from build123d import *

# Parameters (mm, degrees)
F0_W     = 20
F0_H     = 20
F1_DEPTH = 15
F1_TAPER = 3
F2_R     = 2
F4_DEPTH = 3


with BuildPart() as f1:
    # F0 (on Top) → F1 (new body)
    with BuildSketch(Plane.XY):
        with Locations((0.5756109022, 1.4432906293)):
            Rectangle(F0_W, F0_H)
    extrude(amount=F1_DEPTH, taper=F1_TAPER)

    # F2
    f2_edges = [f1.edges().sort_by_distance(p)[0] for p in [
        (10.182552, 11.050232, 7.500009),
        (-9.031331, 11.050232, 7.5),
        (0.575611, 10.657174, 15),
        (9.789494, 1.443291, 15),
        (-8.638272, 1.443291, 15),
        (0.575611, -7.770593, 15),
        (10.182553, -8.163651, 7.5),
        (-9.031331, -8.163651, 7.5),
    ]]
    fillet(f2_edges, radius=F2_R)

    # F3 (on face) → F4 (cut)
    with BuildSketch(Plane.XY.offset(15)):
        with BuildLine():
            ThreePointArc((0.0739849746, 2.8522026186), (0.0610210241, 2.3942139809), (-0.3458335996, 2.1835223306))
            ThreePointArc((-0.3458335996, 2.1835223306), (-1.6651722336, 3.0450533776), (-2.5740938727, 4.332202021))
            ThreePointArc((-2.5740938727, 4.332202021), (-3.2984354247, 4.3375147134), (-3.5025356337, 3.6425024737))
            ThreePointArc((-3.5025356337, 3.6425024737), (-2.2013261333, 1.9150900343), (-0.3458335996, 0.8041231777))
            ThreePointArc((-0.3458335996, 0.8041231777), (-0.1755041632, -1.0493512959), (-0.7172103506, -2.8300629929))
            ThreePointArc((-0.7172103506, -2.8300629929), (-1.3788731625, -4.0087859867), (-2.0861055236, -5.160744302))
            ThreePointArc((-2.0861055236, -5.160744302), (-1.4661125478, -5.5869675362), (-0.7172103506, -5.5148354732))
            ThreePointArc((-0.7172103506, -5.5148354732), (-0.0370124501, -4.6360900284), (0.5756109022, -3.708967939))
            ThreePointArc((0.5756109022, -3.708967939), (1.1882342544, -4.6360900284), (1.8684321549, -5.5148354732))
            ThreePointArc((1.8684321549, -5.5148354732), (2.6173343521, -5.5869675362), (3.237327328, -5.160744302))
            ThreePointArc((3.237327328, -5.160744302), (2.5300949668, -4.0087859867), (1.8684321549, -2.8300629929))
            ThreePointArc((1.8684321549, -2.8300629929), (1.3267259675, -1.0493512959), (1.4970554039, 0.8041231777))
            ThreePointArc((1.4970554039, 0.8041231777), (3.3525479377, 1.9150900343), (4.6537574381, 3.6425024737))
            ThreePointArc((4.6537574381, 3.6425024737), (4.449657229, 4.3375147134), (3.725315677, 4.332202021))
            ThreePointArc((3.725315677, 4.332202021), (2.8163940379, 3.0450533776), (1.4970554039, 2.1835223306))
            ThreePointArc((1.4970554039, 2.1835223306), (1.0790271453, 2.4130070709), (1.100178456, 2.8894139275))
            ThreePointArc((1.100178456, 2.8894139275), (0.4912082686, 5.5147546705), (0.0739849746, 2.8522026186))
        make_face()
    extrude(amount=-F4_DEPTH, mode=Mode.SUBTRACT)


solid = f1.part
Input: part model. Units: mm. Frame: model coordinates. A direction names the side the tool comes from. Coordinates: 2 decimals unless noted, no trailing zeros. Loops run counter-clockwise (first coordinate to the right, second up) from the corner with the lowest first, then second, coordinate; pieces in that order, holes last. Notation, with made-up numbers: (32, 15) -> (70, 15) arc R22 ccw to (70, 33) -> close; hole circle Ø7 at (78.25, -28.75). An arc over 180 degrees is marked (long way). Write item = value, one per line. Start each with the question number.
Item 1: First-contact query: P1, Ø2, axis at x = -2.5, z = 7, coming from the +Y side; P2, Ø8, axis at x = -5, z = 11, coming from the -Y side; P3, Ø3, axis at x = 6, z = 10.5, coming from the -Y side; P4, Ø3.5, axis at x = 0.54, y = 4.14, coming from the +Z side. Flat tips, straight axial feed; report the tip coordinate or a pass-through.
Item 2: Cut plane B-B, the plane x = -3. Return loops of the section in (y, z), plus the area to 3 significant figures.
Item 3: Mould query, pull axis Y, two halves, no side actions, for faces 1 (the face through (1.179, -4.623, 13.521)), 2 (the face through (-8.506, -7.608, 6.657)), 3 (the face through (-1, 3, 15)), 4 (the face through (-3.29, 4.344, 13.521)). Classes: pulls with the +Y half, pulls with the -Y half, needs draft (parallel to the pull), parting line crosses it, or undercut.
Item 4: Cut plane A-A, the plane y = -1.5. Return loops of the section in (x, z).
Item 5: Material intervals for line 1 (X direction, y = -5, z = 12.25); line 2 (X direction, y = -2.5, z = 12.75); line 3 (Z direction, x = 6.5, y = -6), sorted ascending.
Item 6: Reachability of faces 5 (the face through (0, 2, 0)), 6 (the face through (-1.65, 3.03, 13.52)) from +Z, -Z, +X, -X, +Y, -Y: full face, straight path, thin tool, end or side. Return the list, or none.
Item 7: Cut plane C-C, the plane y = 6. Return loops of the section in (x, z), plus the area to 3 significant figures.
Ans:
q1.P1 = 11.13
q1.P2 = -8.19
q1.P3 = -8.09
q1.P4 = 15
q2.outline = (-8.56, 0) -> (11.44, 0) -> (10.76, 13.1) arc R2 ccw to (8.76, 15) -> (4.45, 15) -> (4.45, 12) -> (2.8, 12) -> (2.8, 15) -> (-5.87, 15) arc R2 ccw to (-7.87, 13.1) -> close
q2.area = 282 mm²
q3.face_1 = undercut
q3.face_2 = pulls with the -Y half
q3.face_3 = needs draft
q3.face_4 = undercut
q4.outline = (-9.42, 0) -> (10.58, 0) -> (9.89, 13.1) arc R2 ccw to (7.89, 15) -> (1.39, 15) -> (1.39, 12) -> (-0.24, 12) -> (-0.24, 15) -> (-6.74, 15) arc R2 ccw to (-8.74, 13.1) -> close
q5.line_1 = -8.78 to -1.98, -0.31 to 1.46, 3.13 to 9.93
q5.line_2 = -8.76 to -0.56, 1.71 to 9.91
q5.line_3 = 0 to 15
q6.face_5 = -Z, +X, -X, +Y, -Y
q6.face_6 = +Z
q7.outline = (-9.42, 0) -> (10.58, 0) -> (9.89, 13.1) arc R2 ccw to (7.89, 15) -> (-6.74, 15) arc R2 ccw to (-8.74, 13.1) -> close
q7.area = 287 mm²
